Build history of the part. All positions in model axes, mm. Face numbers are marked on the shaded views. A direction names the side the tool comes from. Give positions to 0.01 mm unless a question says otherwise; leave off trailing zeros. Order: outer loops, then holes, each group sorted by start corner. A loop starts at its lowest first (then second) coordinate and runs counter-clockwise, first axis right, second up. Notation, with made-up numbers: (8, 23) - (65, 23) arc R5 cw to (65, 32) - close; hole circle Ø9 at (37, 82.25). An arc over 180 degrees is marked (long way). Write each question's results on one line, items separated by ' | '. Start each with the question number.
1) Two-plate mould, pull along Y, no slides. Class the marked faces 1, 2, 3 and 4: +Y half, -Y half, draft (parallel to the pull), parting line (faces both ways), or undercut.
2) Drill centre lines: line 1 along Y through (x, z) = (71, -22); line 2 along X through (y, z) = (-5, -29); line 3 along Y through (x, z) = (34.5, -31). Where is each one in solid material? Low to high. Write a range as from..to.
3) Drop flat-ended pins along their axis: pin 1 Ø4 at (x, y) = (93.5, -11.5) entering from -Z; pin 2 Ø8 at (x, y) = (72.33, -44) entering from +Z; pin 3 Ø5 at (y, z) = (-34, -11.5) entering from +X; pin 4 Ø3 at (y, z) = (-42.5, -29) entering from +X. Give the stop position or say it passes through.
4) Cut at A-A on x = 65. List the corners of the cut face in (y, z), plus the area to 3 significant figures.
5) Tool access for the marked faces 5, 6 and 7: list every direction of +Z, -Z, +X, -X, +Y, -Y with a clear straight run to the whole face (end or side of a thin tool).
6) Cut at C-C on x = 46. List the corners of the cut face in (y, z).
7) Cut at B-B on z = -32. List the corners of the cut face in (x, y).
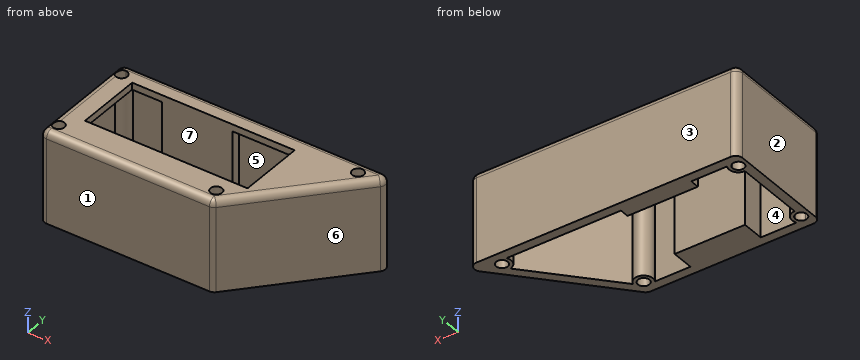
from build123d import *

# Parameters (mm, degrees)
F1_DEPTH     = 3
F0_R         = 2.5
F0_W         = 30.5
F0_H         = 9.5
F0_H_2       = 4
F2_DEPTH     = 39.6
F3_T1_DEPTH  = 70.6639127859
F3_T3_DEPTH  = 44.1
F3_T5_DEPTH  = 39.9402180353
F3_T7_DEPTH  = 59.1959458071
F3_T9_DEPTH  = 53.4402180353
F3_T11_DEPTH = 110.2639127859
F3_T13_DEPTH = 44
F3_S17_W     = 3
F3_S17_H     = 3
F3_T18_DEPTH = 3
F3_T24_DEPTH = 3
F3_T30_DEPTH = 3
F3_S35_W     = 3
F3_S35_H     = 3
F3_T36_DEPTH = 3


# Not quite as in the source:
# - a fillet or chamfer that OpenCascade refuses, or shapes differently, is made with other operations: its cross-section is extruded or revolved along the edge and cut away or added


with BuildPart() as f1:
    # F0 (on Top) → F1 (new body)
    with BuildSketch(Plane.XY):
        with BuildLine():
            Line((10, -36.5), (10, -8))
            Line((10, -8), (23, -8))
            Line((23, -8), (23, -4))
            Line((23, -4), (7.4641016151, -4))
            ThreePointArc((7.4641016151, -4), (7.4641016151, -8), (4, -10))
            Line((4, -10), (4, -40))
            ThreePointArc((4, -40), (7.4641016151, -42), (7.4641016151, -46))
            Line((7.4641016151, -46), (23, -46))
            Line((23, -46), (23, -36.5))
            Line((23, -36.5), (10, -36.5))
        make_face()
    extrude(amount=-F1_DEPTH)



with BuildPart() as f1b:
    # F0 (on Top) → F1, piece 2 (new body)
    with BuildSketch(Plane.XY):
        with BuildLine():
            Line((53.5, -4), (53.5, -8))
            Line((53.5, -8), (80.5, -8))
            Line((80.5, -8), (80.5, -36.5))
            Line((80.5, -36.5), (53.5, -36.5))
            Line((53.5, -36.5), (53.5, -46))
            Line((53.5, -46), (68.8637239566, -46))
            ThreePointArc((68.8637239566, -46), (70.700471232, -40.3459997464), (76.1317756715, -42.7630830107))
            Line((76.1317756715, -42.7630830107), (105.697052057, -9.9127759158))
            ThreePointArc((105.697052057, -9.9127759158), (102.8738253182, -7.6273543397), (103.0637239566, -4))
            Line((103.0637239566, -4), (53.5, -4))
        make_face()
    extrude(amount=-F1_DEPTH)


with BuildPart() as f1_1:
    add(f1.part)

    add(f1b.part)  # F2 merges F1b
    # F0 (on Top) → F2 (join)
    with BuildSketch(Plane.XY):
        Polygon((120, 0), (0, 0), (0, -50), (75, -50), align=None)
        with BuildLine():
            ThreePointArc((4, -46.5), (2.232233047, -42.232233047), (6.5, -44))
            ThreePointArc((6.5, -44), (5.767766953, -45.767766953), (4, -46.5))
        make_face(mode=Mode.SUBTRACT)
        with BuildLine():
            Line((7.4641016151, -4), (23, -4))
            Line((23, -4), (53.5, -4))
            Line((53.5, -4), (103.0637239566, -4))
            ThreePointArc((103.0637239566, -4), (102.8738253182, -7.6273543397), (105.697052057, -9.9127759158))
            Line((105.697052057, -9.9127759158), (76.1317756715, -42.7630830107))
            ThreePointArc((76.1317756715, -42.7630830107), (70.700471232, -40.3459997464), (68.8637239566, -46))
            Line((68.8637239566, -46), (53.5, -46))
            Line((53.5, -46), (23, -46))
            Line((23, -46), (7.4641016151, -46))
            ThreePointArc((7.4641016151, -46), (7.4641016151, -42), (4, -40))
            Line((4, -40), (4, -10))
            ThreePointArc((4, -10), (7.4641016151, -8), (7.4641016151, -4))
        make_face(mode=Mode.SUBTRACT)
        with Locations((72.3278255718, -44)):
            Circle(F0_R, mode=Mode.SUBTRACT)
        with BuildLine():
            ThreePointArc((4, -3.5), (5.767766953, -4.232233047), (6.5, -6))
            ThreePointArc((6.5, -6), (2.232233047, -7.767766953), (4, -3.5))
        make_face(mode=Mode.SUBTRACT)
        with Locations((106.5278255718, -6)):
            Circle(F0_R, mode=Mode.SUBTRACT)
        with Locations((38.25, -41.25)):
            Rectangle(F0_W, F0_H)
        with Locations((38.25, -6)):
            Rectangle(F0_W, F0_H_2)
    extrude(amount=-F2_DEPTH)

    # F3: fillet of radius 3 on 8 edges, made by hand

    # F3_s2 → F3_t1 (cut)
    with BuildSketch(Plane.YZ.offset(3)):
        with BuildLine():
            ThreePointArc((-50, -3), (-49.1213203436, -0.8786796564), (-47, 0))
            Line((-47, 0), (-50, 0))
            Line((-50, 0), (-50, -3))
        make_face()
    extrude(amount=F3_T1_DEPTH, mode=Mode.SUBTRACT)

    # F3_s4 → F3_t3 (cut)
    with BuildSketch(Plane.XY.offset(-47.1)):
        with BuildLine():
            ThreePointArc((3, -50), (0.8786796564, -49.1213203436), (0, -47))
            Line((0, -47), (0, -50))
            Line((0, -50), (3, -50))
        make_face()
        with BuildLine():
            ThreePointArc((0, -3), (0.8786796564, -0.8786796564), (3, 0))
            Line((3, 0), (0, 0))
            Line((0, 0), (0, -3))
        make_face()
    extrude(amount=F3_T3_DEPTH, mode=Mode.SUBTRACT)

    # F3_s6 → F3_t5 (cut)
    with BuildSketch(Plane.XY.offset(-42.9402180353)):
        with BuildLine():
            ThreePointArc((75.8937952246, -49.0068941949), (74.8844285407, -49.7405001902), (73.6639127859, -50))
            Line((73.6639127859, -50), (75, -50))
            Line((75, -50), (75.8937952246, -49.0068941949))
        make_face()
    extrude(amount=F3_T5_DEPTH, mode=Mode.SUBTRACT)

    # F3_s8 → F3_t7 (cut)
    with BuildSketch(Plane(origin=(9.5954526832, 10.6616140924, 0), x_dir=(0, 0, 1), z_dir=(0.6689647316, 0.7432941462, 0))):
        with BuildLine():
            ThreePointArc((-3, 89.1952975497), (-0.8786796564, 88.3166178932), (0, 86.1952975497))
            Line((0, 86.1952975497), (0, 89.1952975497))
            Line((0, 89.1952975497), (-3, 89.1952975497))
        make_face()
    extrude(amount=F3_T7_DEPTH, mode=Mode.SUBTRACT)

    # F3_s10 → F3_t9 (cut)
    with BuildSketch(Plane.XY.offset(-56.4402180353)):
        with BuildLine():
            ThreePointArc((115.4937952246, -5.0068941949), (116.004412976, -1.7794842452), (113.2639127859, 0))
            Line((113.2639127859, 0), (120, 0))
            Line((120, 0), (115.4937952246, -5.0068941949))
        make_face()
    extrude(amount=F3_T9_DEPTH, mode=Mode.SUBTRACT)

    # F3_s12 → F3_t11 (cut)
    with BuildSketch(Plane.YZ.offset(3)):
        with BuildLine():
            ThreePointArc((0, -3), (-0.8786796564, -0.8786796564), (-3, 0))
            Line((-3, 0), (0, 0))
            Line((0, 0), (0, -3))
        make_face()
    extrude(amount=F3_T11_DEPTH, mode=Mode.SUBTRACT)

    # F3_s14 → F3_t13 (cut)
    with BuildSketch(Plane.XZ.offset(3)):
        with BuildLine():
            ThreePointArc((0, -3), (0.8786796564, -0.8786796564), (3, 0))
            Line((3, 0), (0, 0))
            Line((0, 0), (0, -3))
        make_face()
    extrude(amount=F3_T13_DEPTH, mode=Mode.SUBTRACT)


with BuildPart() as f3_tool16:
    # F3_s17 → F3_t18 (new body)
    with BuildSketch(Plane.XY.offset(-3)):
        with Locations((1.5, -48.5)):
            Rectangle(F3_S17_W, F3_S17_H)
    extrude(amount=F3_T18_DEPTH)

    # F3_s19 → F3_t20 (revolve, cut)
    with BuildSketch(Plane(origin=(3, -47, -3), x_dir=(0.7071067812, 0.7071067812, 0), z_dir=(0.7071067812, -0.7071067812, 0))):
        with BuildLine():
            ThreePointArc((0, -3), (3, 0), (0, 3))
            Line((0, 3), (0, -3))
        make_face()
    revolve(axis=Axis((3, -47, -3), (0, 0, 1)), mode=Mode.SUBTRACT)


with BuildPart() as f1_2:
    add(f1_1.part)

    # F3_t15: cut F3_tool16
    add(f3_tool16.part, mode=Mode.SUBTRACT)


with BuildPart() as f3_tool22:
    # F3_s23 → F3_t24 (new body)
    with BuildSketch(Plane.XY.offset(-3)):
        Polygon((73.6639127859, -47), (75.8937952246, -49.0068941949), (75, -50), (73.6639127859, -50), align=None)
    extrude(amount=F3_T24_DEPTH)

    # F3_s25 → F3_t26 (revolve, cut)
    with BuildSketch(Plane(origin=(73.6639127859, -47, -3), x_dir=(-0.4068385849, 0.9135000634, 0), z_dir=(0.9135000634, 0.4068385849, 0))):
        with BuildLine():
            ThreePointArc((0, -3), (3, 0), (0, 3))
            Line((0, 3), (0, -3))
        make_face()
    revolve(axis=Axis((73.6639127859, -47, -3), (0, 0, 1)), mode=Mode.SUBTRACT)


with BuildPart() as f1_3:
    add(f1_2.part)

    # F3_t21: cut F3_tool22
    add(f3_tool22.part, mode=Mode.SUBTRACT)


with BuildPart() as f3_tool28:
    # F3_s29 → F3_t30 (new body)
    with BuildSketch(Plane.XY.offset(-3)):
        Polygon((113.2639127859, -3), (115.4937952246, -5.0068941949), (120, 0), (113.2639127859, 0), align=None)
    extrude(amount=F3_T30_DEPTH)

    # F3_s31 → F3_t32 (revolve, cut)
    with BuildSketch(Plane(origin=(113.2639127859, -3, -3), x_dir=(-0.9135000634, -0.4068385849, 0), z_dir=(-0.4068385849, 0.9135000634, 0))):
        with BuildLine():
            ThreePointArc((0, -3), (3, 0), (0, 3))
            Line((0, 3), (0, -3))
        make_face()
    revolve(axis=Axis((113.2639127859, -3, -3), (0, 0, 1)), mode=Mode.SUBTRACT)


with BuildPart() as f1_4:
    add(f1_3.part)

    # F3_t27: cut F3_tool28
    add(f3_tool28.part, mode=Mode.SUBTRACT)


with BuildPart() as f3_tool34:
    # F3_s35 → F3_t36 (new body)
    with BuildSketch(Plane.XZ.offset(3)):
        with Locations((1.5, -1.5)):
            Rectangle(F3_S35_W, F3_S35_H)
    extrude(amount=-F3_T36_DEPTH)

    # F3_s37 → F3_t38 (revolve, cut)
    with BuildSketch(Plane(origin=(3, -3, -3), x_dir=(0.7071067812, 0, -0.7071067812), z_dir=(0.7071067812, 0, 0.7071067812))):
        with BuildLine():
            ThreePointArc((0, -3), (3, 0), (0, 3))
            Line((0, 3), (0, -3))
        make_face()
    revolve(axis=Axis((3, -3, -3), (0, 1, 0)), mode=Mode.SUBTRACT)


with BuildPart() as f1_5:
    add(f1_4.part)

    # F3_t33: cut F3_tool34
    add(f3_tool34.part, mode=Mode.SUBTRACT)


solid = f1_5.part
Results:
1) face 1: -Y half | face 2: draft | face 3: +Y half | face 4: undercut
2) line 1: -50..-46.12, -41.88..-40.23, -4..0 | line 2: 0..1.71, 6.29..7.87, 23..53.5, 102.65..104.24, 108.82..115.5 | line 3: -50..-36.5, -8..0
3) pin 1: z = -3 | pin 2: z = 0 | pin 3: x = 91.65 | pin 4: x = 83.1
4) outline: (-50, -39.6) - (-46, -39.6) - (-46, -3) - (-36.5, -3) - (-36.5, 0) - (-47, 0) arc R3 ccw to (-50, -3) - close; (-8, -3) - (-4, -3) - (-4, -39.6) - (0, -39.6) - (0, -3) arc R3 ccw to (-3, 0) - (-8, 0) - close | area: 353 mm^2
5) face 5: -Z | face 6: +Z, -Z, +X, -Y | face 7: +Z, -Z
6) outline: (-50, -39.6) - (-36.5, -39.6) - (-36.5, 0) - (-47, 0) arc R3 ccw to (-50, -3) - close; (-8, -39.6) - (0, -39.6) - (0, -3) arc R3 ccw to (-3, 0) - (-8, 0) - close
7) outline: (0, -47) arc R3 ccw to (3, -50) - (73.66, -50) arc R3 ccw to (75.89, -49.01) - (115.49, -5.01) arc R3 ccw to (113.26, 0) - (3, 0) arc R3 ccw to (0, -3) - close; hole circle Ø5 at (4, -44); hole circle Ø5 at (4, -6); hole (4, -40) arc R4 cw to (7.46, -46) - (23, -46) - (23, -36.5) - (53.5, -36.5) - (53.5, -46) - (68.86, -46) arc R4 cw (long way) to (76.13, -42.76) - (105.7, -9.91) arc R4 cw to (103.06, -4) - (53.5, -4) - (53.5, -8) - (23, -8) - (23, -4) - (7.46, -4) arc R4 cw to (4, -10) - close; hole circle Ø5 at (72.33, -44); hole circle Ø5 at (106.53, -6)
